from build123d import *

# Parameters (mm, degrees)
SKETCH1_W           = 50.8
SKETCH1_H           = 50.8
BOSS_EXTRUDE1_DEPTH = 3.175
SKETCH2_R           = 3.175
BOSS_EXTRUDE2_DEPTH = 9.525
SKETCH3_R           = 1.98374
CUT_EXTRUDE1_DEPTH  = 13.7


with BuildPart() as part:
    # Sketch1 → Boss-Extrude1 (new body)
    with BuildSketch(Plane(origin=(0, 0, 0), x_dir=(1, 0, 0), z_dir=(0, 1, 0))):
        Rectangle(SKETCH1_W, SKETCH1_H)
    extrude(amount=BOSS_EXTRUDE1_DEPTH)

    # Sketch2 → Boss-Extrude2 (add)
    with BuildSketch(Plane(origin=(0, 3.175, 0), x_dir=(1, 0, 0), z_dir=(0, 1, 0))):
        with Locations((0, 19.05)):
            Circle(SKETCH2_R)
        with Locations((13.470384182, 13.470384182)):
            Circle(SKETCH2_R)
        with Locations((19.05, 0)):
            Circle(SKETCH2_R)
        with Locations((13.470384182, -13.470384182)):
            Circle(SKETCH2_R)
        with Locations((0, -19.05)):
            Circle(SKETCH2_R)
        with Locations((-13.470384182, -13.470384182)):
            Circle(SKETCH2_R)
        with Locations((-19.05, 0)):
            Circle(SKETCH2_R)
        with Locations((-13.470384182, 13.470384182)):
            Circle(SKETCH2_R)
        Circle(SKETCH2_R)
    extrude(amount=BOSS_EXTRUDE2_DEPTH)

    # Sketch3 → Cut-Extrude1 (cut, through all)
    with BuildSketch(Plane(origin=(0, 12.7, 0), x_dir=(1, 0, 0), z_dir=(0, 1, 0))):
        with Locations((0, 19.05)):
            Circle(SKETCH3_R)
        with Locations((13.470384182, 13.470384182)):
            Circle(SKETCH3_R)
        with Locations((19.05, 0)):
            Circle(SKETCH3_R)
        with Locations((13.470384182, -13.470384182)):
            Circle(SKETCH3_R)
        with Locations((0, -19.05)):
            Circle(SKETCH3_R)
        with Locations((-13.470384182, -13.470384182)):
            Circle(SKETCH3_R)
        with Locations((-19.05, 0)):
            Circle(SKETCH3_R)
        with Locations((-13.470384182, 13.470384182)):
            Circle(SKETCH3_R)
        Circle(SKETCH3_R)
    extrude(amount=-CUT_EXTRUDE1_DEPTH, mode=Mode.SUBTRACT)


solid = part.part
Verification items for the finished model (mm, model axes). A direction names the side the tool comes from. Coordinates: 2 decimals unless noted, no trailing zeros. Order: outer loops, then holes, each group sorted by start corner. A loop starts at its lowest first (then second) coordinate and runs counter-clockwise, first axis right, second up.
Item 1: Section check A-A, the plane z = 0. Enter the section's corners in (x, y) (3 decimals), then the cut area to 3 significant figures.
Filled in:
outline: (-25.4, 0) - (-21.034, 0) - (-21.034, 12.7) - (-22.225, 12.7) - (-22.225, 3.175) - (-25.4, 3.175) - close; (-17.066, 0) - (-1.984, 0) - (-1.984, 12.7) - (-3.175, 12.7) - (-3.175, 3.175) - (-15.875, 3.175) - (-15.875, 12.7) - (-17.066, 12.7) - close; (1.984, 0) - (17.066, 0) - (17.066, 12.7) - (15.875, 12.7) - (15.875, 3.175) - (3.175, 3.175) - (3.175, 12.7) - (1.984, 12.7) - close; (21.034, 0) - (25.4, 0) - (25.4, 3.175) - (22.225, 3.175) - (22.225, 12.7) - (21.034, 12.7) - close
area: 192 mm2
Item 2: Section check C-C, the plane y = 4.5. Give the number of separate pieces and of enclosed holes in the cut face, then the cut area to 3 significant figures.
Filled in:
separate pieces: 9
enclosed holes: 9
area: 174 mm2
Item 3: Release check for a two-part mould opening along X. For faces 1 (the face through (-15, 12.7, 15)), 2 (the face through (17.07, 6.44, -0.09)), 3 (the face through (-25.4, 2, 0)) record: +X half, -X half, draft (parallel to the pull), parting line (faces both ways), or undercut.
Filled in:
face 1: draft
face 2: undercut
face 3: -X half
Item 4: Access from +Z, -Z, +X, -X, +Y, -Y to the whole of each face (thin tool, end or side, straight path). Record for faces 4 (the face through (0, 2, 25.4)), 5 (the face through (3.03, 7.87, 18.1)).
Filled in:
face 4: +Z, +X, -X, +Y, -Y
face 5: +Y
Item 5: Section check D-D, the plane z = 14.5. Enter the section's corners in (x, y) (3 decimals), then the cut area to 3 significant figures.
Filled in:
outline: (-25.4, 0) - (-15.166, 0) - (-15.166, 12.7) - (-16.474, 12.7) - (-16.474, 3.175) - (-25.4, 3.175) - close; (-11.775, 0) - (11.775, 0) - (11.775, 12.7) - (10.467, 12.7) - (10.467, 3.175) - (-10.467, 3.175) - (-10.467, 12.7) - (-11.775, 12.7) - close; (15.166, 0) - (25.4, 0) - (25.4, 3.175) - (16.474, 3.175) - (16.474, 12.7) - (15.166, 12.7) - close
area: 190 mm2
Item 6: Section check B-B, the plane x = 0. Enter the section's corners in (y, z) (3 decimals), then the cut area to 3 significant figures.
Filled in:
outline: (0, -25.4) - (3.175, -25.4) - (3.175, -22.225) - (12.7, -22.225) - (12.7, -21.034) - (0, -21.034) - close; (0, -17.066) - (12.7, -17.066) - (12.7, -15.875) - (3.175, -15.875) - (3.175, -3.175) - (12.7, -3.175) - (12.7, -1.984) - (0, -1.984) - close; (0, 1.984) - (12.7, 1.984) - (12.7, 3.175) - (3.175, 3.175) - (3.175, 15.875) - (12.7, 15.875) - (12.7, 17.066) - (0, 17.066) - close; (0, 21.034) - (12.7, 21.034) - (12.7, 22.225) - (3.175, 22.225) - (3.175, 25.4) - (0, 25.4) - close
area: 192 mm2
Item 7: Material ranges on L1, parallel to X at y = 7.25, z = 0 (3 decimals); L2, parallel to Z at x = 1.5, y = 5.25, recorded low to high.
Filled in:
L1: x = -22.225 to -21.034, -17.066 to -15.875, -3.175 to -1.984, 1.984 to 3.175, 15.875 to 17.066, 21.034 to 22.225
L2: z = -21.85 to -20.35, -17.75 to -16.25, -2.8 to -1.3, 1.3 to 2.8, 16.25 to 17.75, 20.35 to 21.85
Item 8: Depth check by flat-ended pin: pin 1 (4 mm diameter, centred on y = 7.5, z = -20, fed in from -X) (3 decimals); pin 2 (3 mm diameter, centred on x = 0, z = -19.05, fed in from -Y); pin 3 (4 mm diameter, centred on x = -12.5, z = -3, fed in from +Y) (3 decimals); pin 4 (5 mm diameter, centred on x = -11, y = 11.5, fed in from +Z). Enter the tip coordinate at first touch or a pass-through.
Filled in:
pin 1: stops at x = -3.175
pin 2: passes through
pin 3: stops at y = 3.175
pin 4: stops at z = 16.65
